Design review of the part built by this model. Coordinates are the model's own, in mm. A direction names the side the tool comes from. Coordinates: 2 decimals unless noted, no trailing zeros. Write each loop counter-clockwise with the first axis right and the second up, starting at its lowest first coordinate (ties: lowest second). Pieces come first, ordered by that corner, then holes. Notation, with made-up numbers: (-36.5, -36.5) - (-13.5, -36.5) arc R12 cw to (-13.5, -25.5) - close; hole circle Ø1 at (8.5, 14). An arc over 180 degrees is marked (long way). Answer as a JSON object with one key per item and string values.
```python
from build123d import *

# Parameters (mm, degrees)
F1_DEPTH = 10


with BuildPart() as f1:
    # F0 (on Top) → F1 (new body)
    with BuildSketch(Plane.XY):
        with BuildLine():
            ThreePointArc((2.5, 4.5596052461), (4.4743714642, 2.6495282599), (5.2, 0))
            ThreePointArc((5.2, 0), (-2.6495282599, -4.4743714642), (-2.5, 4.5596052461))
            Line((-2.5, 4.5596052461), (-2.5, 6.7520367298))
            ThreePointArc((-2.5, 6.7520367298), (-4.1133927602, -5.9093146811), (7.2, 0))
            ThreePointArc((7.2, 0), (5.9093146811, 4.1133927602), (2.5, 6.7520367298))
            Line((2.5, 6.7520367298), (2.5, 4.5596052461))
        make_face()
        with BuildLine():
            ThreePointArc((-4.53e-08, 7.2), (1.2699085464, 7.0871244016), (2.5, 6.7520367298))
            Line((2.5, 6.7520367298), (2.5, 7.5348486101))
            ThreePointArc((2.5, 7.5348486101), (1.261162496, 7.2840842634), (-4.53e-08, 7.2))
        make_face()
        with BuildLine():
            Line((-2.5, 7.5348486101), (-2.5, 6.7520367298))
            ThreePointArc((-2.5, 6.7520367298), (-1.269908591, 7.0871243936), (-4.53e-08, 7.2))
            ThreePointArc((-4.53e-08, 7.2), (-1.2611625409, 7.2840842694), (-2.5, 7.5348486101))
        make_face()
        with BuildLine():
            Line((2.5, 9.6289321881), (2.5, 7.5348486101))
            ThreePointArc((2.5, 7.5348486101), (7.5498344353, 10.9337187027), (9.5, 16.7))
            ThreePointArc((9.5, 16.7), (8.0122187352, 21.8043462793), (4.0148734865, 25.3099239768))
            Line((4.0148734865, 25.3099239768), (3.1696369631, 23.4973084028))
            ThreePointArc((3.1696369631, 23.4973084028), (6.3254358436, 20.7297470626), (7.5, 16.7))
            ThreePointArc((7.5, 16.7), (6.123724357, 12.3698729811), (2.5, 9.6289321881))
        make_face()
        with BuildLine():
            ThreePointArc((-2.5, 4.5596052461), (0, 5.2), (2.5, 4.5596052461))
            Line((2.5, 4.5596052461), (2.5, 6.7520367298))
            ThreePointArc((2.5, 6.7520367298), (1.2699085464, 7.0871244016), (-4.53e-08, 7.2))
            ThreePointArc((-4.53e-08, 7.2), (-1.269908591, 7.0871243936), (-2.5, 6.7520367298))
            Line((-2.5, 6.7520367298), (-2.5, 4.5596052461))
        make_face()
        with BuildLine():
            ThreePointArc((-2.5, 7.5348486101), (-1.2611625409, 7.2840842694), (-4.53e-08, 7.2))
            ThreePointArc((-4.53e-08, 7.2), (1.261162496, 7.2840842634), (2.5, 7.5348486101))
            Line((2.5, 7.5348486101), (2.5, 9.6289321881))
            ThreePointArc((2.5, 9.6289321881), (0, 9.2), (-2.5, 9.6289321881))
            Line((-2.5, 9.6289321881), (-2.5, 7.5348486101))
        make_face()
        with BuildLine():
            ThreePointArc((-4.0148734865, 25.3099239768), (-9.4656864627, 15.8932907648), (-2.5, 7.5348486101))
            Line((-2.5, 7.5348486101), (-2.5, 9.6289321881))
            ThreePointArc((-2.5, 9.6289321881), (-7.4912722905, 16.3382826116), (-3.1696369631, 23.4973084028))
            Line((-3.1696369631, 23.4973084028), (-4.0148734865, 25.3099239768))
        make_face()
    extrude(amount=F1_DEPTH)


solid = f1.part
```
(1) For pin 1 (0.9 mm diameter, centred on y = 7, z = 3.5, fed in from +X); pin 2 (8.5 mm diameter, centred on x = 0, y = 0, fed in from +Z); pin 3 (0.9 mm diameter, centred on y = 7, z = 7, fed in from -X); pin 4 (3 mm diameter, centred on x = 3, z = 5.5, fed in from -Y), all flat-tipped, find the tip position at first contact; note any pin that passes through.
Solved:
{"pin 1": "stops at x = 2.99", "pin 2": "passes through", "pin 3": "stops at x = -2.99", "pin 4": "stops at y = -7.04"}
(2) Take a section at C-C, the plane y = 1. Write out the cut boundary in (x, z).
Solved:
{"outline": "(-7.13, 0) - (-5.1, 0) - (-5.1, 10) - (-7.13, 10) - close; (5.1, 0) - (7.13, 0) - (7.13, 10) - (5.1, 10) - close"}
(3) Take a section at B-B, the plane z = 1.5. Write out the cut boundary in (x, y), and give its area (3 significant figures).
Solved:
{"outline": "(-4.01, 25.31) arc R9.5 ccw to (-2.5, 7.53) - (-2.5, 6.75) arc R7.2 ccw (long way) to (2.5, 6.75) - (2.5, 7.53) arc R9.5 ccw to (4.01, 25.31) - (3.17, 23.5) arc R7.5 cw (long way) to (-3.17, 23.5) - close; hole circle Ø10.4 at (0, 0)", "area": "171 mm^2"}
(4) The part is to be moulded in two halves that separate along Y. For faces 3 (the face through (-1, 8, 10)), 4 (the face through (3.6, 24.42, 4.93)), 5 (the face through (-9.48, 16.06, 4.93)), say which applies: pulls with the +Y half, pulls with the -Y half, needs draft (parallel to the pull), parting line crosses it, or undercut.
Solved:
{"face 3": "needs draft", "face 4": "pulls with the +Y half", "face 5": "undercut"}
(5) To check wall thickness, follow line 1 (X direction, y = 0, z = 4.5); line 2 (Y direction, x = 3, z = 4); line 3 (X direction, y = 10, z = 5.75). State the ranges of each line that lie inside material, in increasing order. Write a range as from..to.
Solved:
{"line 1": "x = -7.2..-5.2, 5.2..7.2", "line 2": "y = -6.55..-4.25, 4.25..6.55, 7.69..9.83", "line 3": "x = -6.73..-3.37, 3.37..6.73"}
(6) Tool access review of faces 1 (the face through (-1, 8, 0)), 2 (the face through (-3.586, 24.391, 4.93)): name each direction out of +Z, -Z, +X, -X, +Y, -Y from which nothing blocks a thin tool from reaching the whole face with its end or side.
Solved:
{"face 1": "-Z, +X, -X, +Y, -Y", "face 2": "+Z, -Z, +Y"}
(7) Take a section at A-A, the plane x = 0. Write out the cut boundary in (y, z), and give its area (3 significant figures).
Solved:
{"outline": "(-7.2, 0) - (-5.2, 0) - (-5.2, 10) - (-7.2, 10) - close; (5.2, 0) - (9.2, 0) - (9.2, 10) - (5.2, 10) - close", "area": "60.0 mm^2"}
(8) Take a section at D-D, the plane x = -6.5. Write out the cut boundary in (y, z), and give its area (3 significant figures).
Solved:
{"outline": "(-3.1, 0) - (3.1, 0) - (3.1, 10) - (-3.1, 10) - close; (9.77, 0) - (12.96, 0) - (12.96, 10) - (9.77, 10) - close; (20.44, 0) - (23.63, 0) - (23.63, 10) - (20.44, 10) - close", "area": "126 mm^2"}
